Build history of the part. All positions in model axes, mm. Face numbers are marked on the shaded views. A direction names the side the tool comes from. Round coordinates to 2 decimals unless told otherwise and drop trailing zeros. Loops run counter-clockwise (first coordinate to the right, second up) from the corner with the lowest first, then second, coordinate; pieces in that order, holes last. Notation, with made-up numbers: (-20, -36.5) -> (10, -36.5) arc R26 ccw to (10, 0.5) -> close; hole circle Ø8 at (34.25, 60.5). An arc over 180 degrees is marked (long way). Put each result on its own line as item: value. Start each with the question number.
Item 1: Flat gauge pins, fed straight in: pin 1 Ø1 at (x, y) = (4.5, 3) entering from +Z; pin 2 Ø0.8 at (x, y) = (43.5, -4) entering from -Z; pin 3 Ø1 at (y, z) = (-13, 25.5) entering from -X. Where does each tip first touch, or does it go through?
Item 2: Drill centre lines: probe 1 along X at (y, z) = (-0.5, 37); probe 2 along Y at (x, z) = (5.5, 10); probe 3 along Z at (x, y) = (-27, -11.5). Where is each one in solid material? Low to high. Write a range as [from, to].
Item 3: Cut at D-D, the plane z = 22. List the corners of the cut face in (x, y), plus the area to 3 significant figures.
Item 4: Cut at B-B, the plane y = -12.5. List the corners of the cut face in (x, z), plus the area to 4 significant figures.
Item 5: Pull direction Y, two halves, no side cores. Call the marked faces 1, 2 and 3: +Y half, -Y half, draft (parallel to the pull), parting line (faces both ways), or undercut.
Item 6: Cut at A-A, the plane z = 7. List the corners of the cut face in (x, y).
Item 7: Cut at C-C, the plane x = -27. List the corners of the cut face in (y, z).
Item 8: Tool access for the marked faces 4 and 5: list every direction of +Z, -Z, +X, -X, +Y, -Y with a clear straight run to the whole face (end or side of a thin tool).
```python
from build123d import *

# Parameters (mm, degrees)
F0_W     = 90
F0_H     = 70
F1_DEPTH = 47.5
F2_T     = -2.5
F3_W     = 30
F3_H     = 17.5
F4_DEPTH = 90


with BuildPart() as f1:
    # F0 (on Top) → F1 (new body)
    with BuildSketch(Plane.XY):
        Rectangle(F0_W, F0_H)
    extrude(amount=F1_DEPTH)

    # F2
    f2_openings = [f1.faces().sort_by_distance(p)[0] for p in [
        (0, 0, 47.5),
    ]]
    offset(amount=F2_T, openings=f2_openings)

    # F3 (on face) → F4 (cut, through all)
    with BuildSketch(Plane.YZ.offset(45)):
        with Locations((0, 23.75)):
            Rectangle(F3_W, F3_H)
    extrude(amount=-F4_DEPTH, mode=Mode.SUBTRACT)


solid = f1.part
```
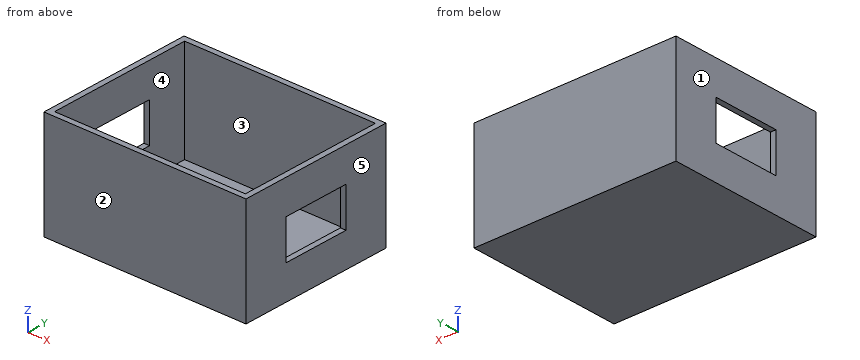
Reply:
1. pin 1: stops at z = 2.5
1. pin 2: stops at z = 0
1. pin 3: passes through
2. probe 1: x = [-45, -42.5], [42.5, 45]
2. probe 2: y = [-35, -32.5], [32.5, 35]
2. probe 3: z = [0, 2.5]
3. outline: (-45, -35) -> (45, -35) -> (45, -15) -> (42.5, -15) -> (42.5, -32.5) -> (-42.5, -32.5) -> (-42.5, -15) -> (-45, -15) -> close; (-45, 15) -> (-42.5, 15) -> (-42.5, 32.5) -> (42.5, 32.5) -> (42.5, 15) -> (45, 15) -> (45, 35) -> (-45, 35) -> close
3. area: 625 mm^2
4. outline: (-45, 0) -> (45, 0) -> (45, 15) -> (42.5, 15) -> (42.5, 2.5) -> (-42.5, 2.5) -> (-42.5, 15) -> (-45, 15) -> close; (-45, 32.5) -> (-42.5, 32.5) -> (-42.5, 47.5) -> (-45, 47.5) -> close; (42.5, 32.5) -> (45, 32.5) -> (45, 47.5) -> (42.5, 47.5) -> close
4. area: 362.5 mm^2
5. face 1: draft
5. face 2: -Y half
5. face 3: undercut
6. outline: (-45, -35) -> (45, -35) -> (45, 35) -> (-45, 35) -> close; hole (-42.5, -32.5) -> (42.5, -32.5) -> (42.5, 32.5) -> (-42.5, 32.5) -> close
7. outline: (-35, 0) -> (35, 0) -> (35, 47.5) -> (32.5, 47.5) -> (32.5, 2.5) -> (-32.5, 2.5) -> (-32.5, 47.5) -> (-35, 47.5) -> close
8. face 4: +Z
8. face 5: +Z, -Z, +X, +Y, -Y
